Solid Edge part; units mm, degrees
sketch "Sketch1" plane through (0, 0, 0) normal (0, 0, 1) x (1, 0, 0)
  line L0 (-11.5, -5) -> (11.5, -5)
  line L1 (11.5, -5) -> (11.5, 5)
  line L2 (11.5, 5) -> (-11.5, 5)
  line L3 (-17.5, 5) -> (-11.5, 5)
  line L4 (-17.5, -1) -> (-17.5, 5)
  line L5 (-17.5, -5) -> (-17.5, -1)
  line L6 (-11.5, -5) -> (-17.5, -5)
extrude "Protrusion1" add sketch "Sketch1" against normal blind 2
sketch "Sketch2" plane through (0, 0, 0) normal (0, 0, 1) x (1, 0, 0)
  circle A0 centre (-14.5, 2) radius 1.5
  circle A1 centre (8.5, 2) radius 1.5
extrude "ExtrudedCutout_1" cut sketch "Sketch2" along normal mid plane 28.6667
sketch "Sketch3" plane through (0, 0, 0) normal (0, 0, 1) x (1, 0, 0)
  line L0 (11.5, 7) -> (-17.5, 7)
  line L1 (-17.5, 7) -> (-17.5, 5)
  line L2 (-17.5, 5) -> (11.5, 5)
  line L3 (11.5, 5) -> (11.5, 7)
extrude "ExtrudedProtrusion_3" add sketch "Sketch3" against normal up to vertex (2 mm away) and the other way blind 13
For this review, take the finished solid that the model builds, in its own axes (mm). A direction names the side the tool comes from. Round coordinates to 2 decimals unless told otherwise and drop trailing zeros. Write each loop counter-clockwise with the first axis right and the second up, starting at its lowest first coordinate (ties: lowest second). Pieces come first, ordered by that corner, then holes. Notation, with made-up numbers: (65, 36.25) - (99, 36.25) arc R35 cw to (99, 68.25) - close; hole circle Ø1 at (58, 42.25). An arc over 180 degrees is marked (long way). Answer as a JSON object with one key per item and string values.
1. Tool access review of faces 1 (the face through (-3, 0, 0)), 2 (the face through (-3, 1, -2)): name each direction out of +Z, -Z, +X, -X, +Y, -Y from which nothing blocks a thin tool from reaching the whole face with its end or side.
Response values:
{"face 1": "+Z, +X, -X, -Y", "face 2": "-Z, +X, -X, +Y, -Y"}
2. We need section B-B on x = -14.5. Give the boundary of the cut face in (y, z), then the cut area to 3 significant figures.
Response values:
{"outline": "(-5, -2) - (0.5, -2) - (0.5, 0) - (-5, 0) - close; (3.5, -2) - (7, -2) - (7, 13) - (5, 13) - (5, 0) - (3.5, 0) - close", "area": "44.0 mm2"}
3. To check wall thickness, follow line 1 along Y through (x, z) = (-14.5, -1.35); line 2 along Z through (x, y) = (-4, -3); line 3 along Y through (x, z) = (-10.5, 6). State the ranges of each line that lie inside material, in increasing order.
Response values:
{"line 1": "y = -5 to 0.5, 3.5 to 7", "line 2": "z = -2 to 0", "line 3": "y = 5 to 7"}
4. We need section C-C on x = -2.25. Give the boundary of the cut face in (y, z).
Response values:
{"outline": "(-5, -2) - (7, -2) - (7, 13) - (5, 13) - (5, 0) - (-5, 0) - close"}
5. We need section D-D on z = 12. Give the boundary of the cut face in (x, y).
Response values:
{"outline": "(-17.5, 5) - (11.5, 5) - (11.5, 7) - (-17.5, 7) - close"}
6. We need section A-A on y = 2. Give the boundary of the cut face in (x, z), then the cut area to 3 significant figures.
Response values:
{"outline": "(-17.5, -2) - (-16, -2) - (-16, 0) - (-17.5, 0) - close; (-13, -2) - (7, -2) - (7, 0) - (-13, 0) - close; (10, -2) - (11.5, -2) - (11.5, 0) - (10, 0) - close", "area": "46.0 mm2"}
7. For pin 1 Ø3.5 at (x, y) = (8.5, 2) entering from +Z; pin 2 Ø5 at (y, z) = (2, 6.5) entering from -X; pin 3 Ø4 at (x, z) = (0, 6.5) entering from -Y, all flat-tipped, find the tip position at first contact; note any pin that passes through.
Response values:
{"pin 1": "stops at z = 0", "pin 2": "passes through", "pin 3": "stops at y = 5"}
8. Draft analysis for pull direction Y (two halves, no side actions). For faces 3 (the face through (11.5, 5.4, 2.8)), 4 (the face through (-3, 7, 6)), 5 (the face through (-16, 2, -1)), state which applies: +Y half, -Y half, draft (parallel to the pull), parting line (faces both ways), or undercut.
Response values:
{"face 3": "draft", "face 4": "+Y half", "face 5": "undercut"}
